Read the model definition and answer for the solid it produces. Units are mm, in the model's axes. A direction names the side the tool comes from. Coordinates: 2 decimals unless noted, no trailing zeros. Order: outer loops, then holes, each group sorted by start corner. A loop starts at its lowest first (then second) coordinate and runs counter-clockwise, first axis right, second up. Notation, with made-up numbers: M 38,-20 L 97,-20 A28 cw 97,14 Z; hole C -25,59.5 d4. An arc over 180 degrees is marked long. Write each question's results on one line, items separated by ' | '.
Autodesk Inventor part; units mm, degrees
ref_plane "Work Plane5" through (-45.25, 188.3183, 3.0535) normal (0, -1, 0) x (1, 0, 0)
ref_plane "YZ Plane" through (0, 0, 0) normal (1, 0, 0) x (0, 1, 0)
ref_plane "XZ Plane" through (0, 0, 0) normal (0, 1, 0) x (-1, 0, 0)
ref_plane "Work Plane4" through (-45.25, 257.5287, -0.5) normal (1, 0, 0) x (0, -1, 0)
sketch "Sketch5" plane through (-45.25, 257.5287, -0.5) normal (1, 0, 0) x (0, -1, 0)
  line L0 (45.7104, -25.5535) -> (92.7104, -25.5535)
  line L1 (92.7104, -25.5535) -> (92.7104, -0.0535)
  line L2 (45.7104, -0.0535) -> (45.7104, -25.5535)
  line L3 (95.2104, -28.0535) -> (43.2104, -28.0535)
  line L4 (43.2104, -28.0535) -> (43.2104, -3.5535)
  line L5 (103.2104, -0.0535) -> (103.2104, -3.5535)
  line L6 (103.2104, -3.5535) -> (95.2104, -3.5535)
  line L7 (92.7104, -0.0535) -> (103.2104, -0.0535)
  line L8 (95.2104, -3.5535) -> (95.2104, -28.0535)
  line L9 (43.2104, -3.5535) -> (35.2104, -3.5535)
  line L10 (35.2104, -3.5535) -> (35.2104, -0.0535)
  line L11 (45.7104, -0.0535) -> (35.2104, -0.0535)
  point P0 (257.5287, -0.5)
  dimension "d10" = 2.5
  dimension "d11" = 3.5
  dimension "d12" = 2.5
  dimension "d13" = 8
  dimension "d14" = 2.5
  dimension "d17" = 8
  dimension "d40" = 47
  dimension "d41" = 25.5
extrude "Extrusion2" add sketch "Sketch5" against normal blind 10
sketch "Sketch6" plane through (-45.25, 154.3183, 3.0535) normal (0, 0, 1) x (1, 0, 0)
  line L0 (0, 68) -> (0, 60)
  line L1 (0, 68) -> (-10, 68)
  line L2 (-10, 60) -> (-10, 68)
  line L3 (0, 60) -> (-10, 60)
  line L4 (0, 8) -> (0, 0)
  line L5 (0, 8) -> (-10, 8)
  line L6 (-10, 0) -> (-10, 8)
  line L7 (0, 0) -> (-10, 0)
  line L8 (-10, 68) -> (0, 60) construction
  line L9 (0, 68) -> (-10, 60) construction
  line L10 (0, 8) -> (-10, 8) construction
  line L11 (-10, 8) -> (0, 0) construction
  line L12 (0, 8) -> (-10, 0) construction
  point P0 (45.25, -154.3183)
  point P1 (-5, 64)
  point P2 (-5, 4)
hole "Hole1" at (-50.25, 218.3183, 3.0535) at (-50.25, 158.3183, 3.0535) direction (0, 0, -1) diameter 3.2 end through all countersink diameter 6 countersink angle 90
sketch "Sketch7" plane through (-55.25, 257.5287, -0.5) normal (-1, 0, 0) x (0, 0, 1)
  line L0 (37.6535, -68.1104) -> (35.0535, -68.1104)
  line L1 (35.0535, -68.1104) -> (35.0535, -70.3104)
  line L2 (35.0535, -70.3104) -> (37.6535, -70.3104)
  line L3 (37.6535, -70.3104) -> (37.6535, -96.3604)
  line L4 (37.6535, -96.3604) -> (28.0535, -96.3604)
  line L5 (28.0535, -96.3604) -> (28.0535, -42.0604)
  line L6 (37.6535, -42.0604) -> (28.0535, -42.0604) construction
  line L7 (37.6535, -42.0604) -> (37.6535, -68.1104) construction
  line L8 (37.6535, -44.5604) -> (40.6535, -44.5604)
  line L9 (40.6535, -44.5604) -> (40.6535, -39.5604)
  line L10 (40.6535, -39.5604) -> (26.6535, -39.5604)
  line L11 (26.6535, -39.5604) -> (24.4035, -43.2104)
  line L12 (3.5535, -43.2104) -> (28.0535, -43.2104)
  line L13 (28.0535, -43.2104) -> (24.4035, -43.2104)
  line L14 (37.8535, -44.5604) -> (37.8535, -41.8604)
  line L15 (37.8535, -41.8604) -> (28.0535, -41.8604)
  line L16 (28.0535, -41.8604) -> (28.0535, -42.0604)
  point P0 (0.5, -257.5287)
  dimension "d42" = 2.5
  dimension "d43" = 3
  dimension "d44" = 5
  dimension "d45" = 3.65
  dimension "d46" = 14
  dimension "d47" = 9.6
  dimension "d48" = 3.65
  dimension "d49" = 0.2
  dimension "d50" = 0.2
extrude "Extrusion3" add sketch "Sketch7" against normal blind 10
chamfer "Chamfer1" distance 4 distance2 2.8 1 edges at (-50.25, 212.9683, 40.1535) measured on face at (-51.9167, 214.6349, 40.1535)
fillet "Fillet2" radius 0.3 2 edges at (-50.25, 212.9683, 37.3536) (-50.25, 212.9683, 37.3535)
ref_plane "Work Plane5" through (-45.25, 188.3183, 3.0535) normal (0, -1, 0) x (1, 0, 0)
mirror "Mirror2" about plane through (-45.25, 188.3183, 3.0535) normal (0, -1, 0) of "Extrusion3", "Fillet2", "Chamfer1"
sketch "Sketch8" plane through (-45.25, 257.5287, -0.5) normal (1, 0, 0) x (0, 0, -1)
  line L0 (-25.5535, -45.7104) -> (-0.0535, -45.7104)
  line L1 (-25.5535, -45.7104) -> (-0.0535, -45.7104)
  line L2 (-0.0535, -45.7104) -> (-0.0535, -45.5104)
  line L3 (-0.0535, -45.5104) -> (-25.5535, -45.5104)
  line L4 (-25.5535, -45.5104) -> (-25.5535, -45.7104)
  line L5 (-0.0535, -92.7104) -> (-25.5535, -92.7104)
  line L6 (-25.5535, -92.7104) -> (-0.0535, -92.7104)
  line L7 (-0.0535, -92.7104) -> (-0.0535, -92.9104)
  line L8 (-0.0535, -92.9104) -> (-25.5535, -92.9104)
  line L9 (-25.5535, -92.9104) -> (-25.5535, -92.7104)
  point P0 (-0.5, -257.5287)
  dimension "d51" = 0.2
  dimension "d52" = 0.2
extrude "Extrusion4" cut sketch "Sketch8" against normal through all
fillet "Fillet3" radius 2 4 edges at (-50.25, 217.9683, 26.1535) (-50.25, 214.3183, 23.9035) (-50.25, 158.6683, 26.1535) (-50.25, 162.3183, 23.9035)
equation "\"d12\" = d10"
equation "\"d14\" = d10"
equation "\"d17\" = d13"
equation "\"d45\" = d48"
properties part number "batteryHolder"
(1) The part is cut by section B-B, the plane x = -50.25. Count the separate pieces of the cut face and the enclosed holes in it, then the cut area to 3 significant figures.
Conclusion:
separate pieces: 3 | enclosed holes: 0 | area: 357 mm²
(2) The part is cut by section C-C, the plane y = 194. Write down the section's boundary in (x, z).
Conclusion:
outline: M -55.25,25.05 L -45.25,25.05 L -45.25,27.55 L -55.25,27.55 Z
(3) Straight lines are drawn through the part: line 1 (Y direction, x = -50.25, z = 0.9); line 2 (Y direction, x = -53, z = 35); line 3 (Z direction, x = -50.5, y = 215). For each, find the intervals that lie inside material, in ascending order.
Conclusion:
line 1: 154.32 to 156.72, 159.92 to 164.62, 212.02 to 216.72, 219.92 to 222.32 | line 2: 158.67 to 160.97, 215.67 to 217.97 | line 3: -0.45 to 3.05, 24.29 to 27.55, 37.35 to 38.78
(4) Given pin 1 (5 mm diameter, centred on x = -54, y = 178.5, fed in from -Z); pin 2 (5 mm diameter, centred on x = -52.5, z = 34.5, fed in from +Y); pin 3 (5 mm diameter, centred on x = -49.5, z = 18, fed in from +Y), each flat-ended and moving along its own axis, determine where each tip first touches the part or whether it passes through.
Conclusion:
pin 1: z = 25.05 | pin 2: y = 217.97 | pin 3: y = 214.32
(5) The mould has two halves that part along Z. Classify faces 1 (the flat face through (-50, 164.618, 12)), 2 (the cylindrical face through (-50.18, 214.579, 23.774)), 3 (the flat face through (-50, 216, -0.446)): pulls with the +Z half, pulls with the -Z half, needs draft (parallel to the pull), parting line crosses it, or undercut.
Conclusion:
face 1: needs draft | face 2: undercut | face 3: pulls with the -Z half
(6) The part is cut by section A-A, the plane z = 33.5. Write down the section's boundary in (x, y).
Conclusion:
outline: M -55.25,158.67 L -45.25,158.67 L -45.25,160.97 L -55.25,160.97 Z; M -55.25,215.67 L -45.25,215.67 L -45.25,217.97 L -55.25,217.97 Z
(7) For faces 4 (the flat face through (-50, 160.968, 32)), 5 (the flat face through (-47, 158, 3.054)), 6 (the cylindrical face through (-50.18, 217.708, 26.283)), 7 (the flat face through (-50, 158.668, 34)), determine the directions among +Z, -Z, +X, -X, +Y, -Y from which every point of the face is accessible in a straight line to the end or side of a thin tool.
Conclusion:
face 4: +X, -X | face 5: +X, -X, -Y | face 6: +X, -X, +Y | face 7: +Z, +X, -X, -Y
